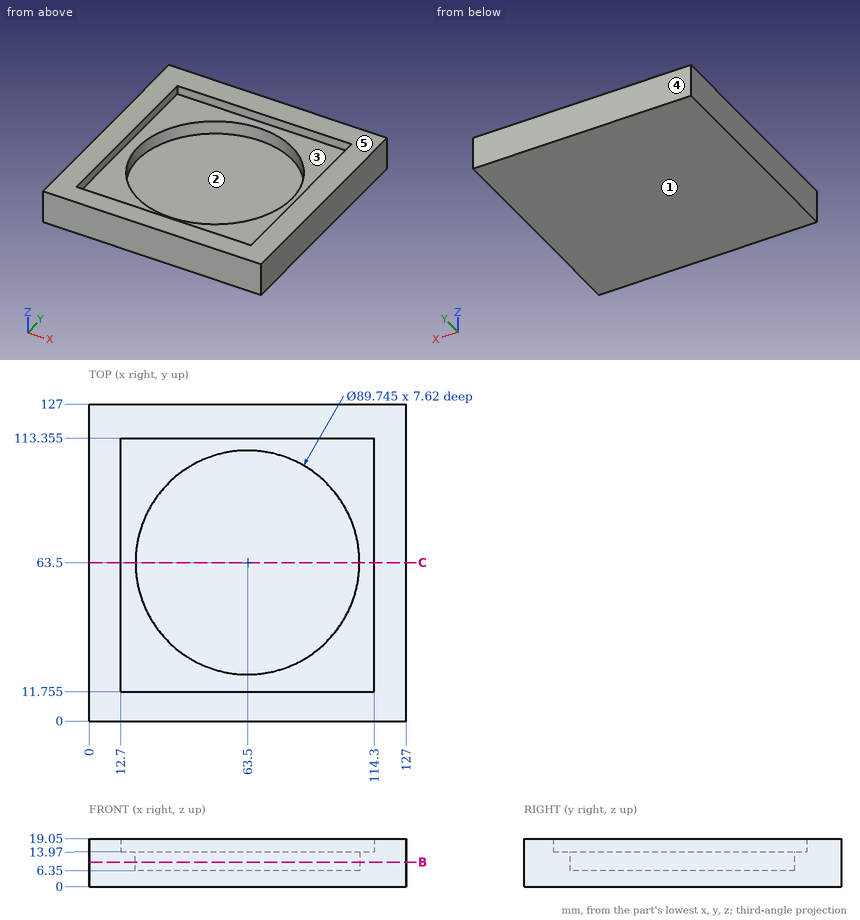
Answer from the drawing. Dimensions are ordinates in mm from the lowest x, y and z of the part. A direction names the side the tool comes from. Coordinates: 2 decimals unless noted, no trailing zeros. Write each loop counter-clockwise with the first axis right and the second up, starting at its lowest first coordinate (ties: lowest second). Pieces come first, ordered by that corner, then holes. Notation, with made-up numbers: (18.25, 33.25) - (27.25, 33.25) arc R32 ccw to (27.25, 60.25) - close; hole circle Ø8 at (41, -38.5). An arc over 180 degrees is marked (long way). Answer as CSV lines item,"result".
1. Find section B-B (z = 9.75). Give the vertices of the cut face in (x, y) (1 decimal).
Computed values:
outline,"(0, 0) - (127, 0) - (127, 127) - (0, 127) - close; hole circle Ø89.7 at (63.5, 63.5)"
2. Find section C-C (y = 63.5). Give the vertices of the cut face in (x, z), plus the area to 3 significant figures.
Computed values:
outline,"(0, 0) - (127, 0) - (127, 19.05) - (114.3, 19.05) - (114.3, 13.97) - (108.37, 13.97) - (108.37, 6.35) - (18.63, 6.35) - (18.63, 13.97) - (12.7, 13.97) - (12.7, 19.05) - (0, 19.05) - close"
area,"1,220 mm²"
3. A tool of negligible diameter and unlimited length cuts with its end or side. For the marked faces 1 and 2, from which of +Z, -Z, +X, -X, +Y, -Y can it reach the whole face along a straight path? Write none if from no direction.
Computed values:
face 1,"-Z, +X, -X, +Y, -Y"
face 2,"+Z"
4. Given P1, Ø2, axis at x = 41, y = 66.5, coming from the -Z side, flat-ended and moving along its own axis, determine where the tip first touches the part or whether it passes through.
Computed values:
P1,"stops at z = 0"
5. Determine the mould class of the marked faces 3, 4 and 5 for opening direction Y: +Y half, -Y half, draft (parallel to the pull), parting line (faces both ways), or undercut.
Computed values:
face 3,"undercut"
face 4,"+Y half"
face 5,"draft"
6. Straight lines are drawn through the part: line 1 (Y direction, x = 79.5, z = 17.75) (1 decimal); line 2 (X direction, y = 92, z = 15.5); line 3 (Z direction, x = 61, y = 24). For each, find the intervals that lie inside material, in ascending order. Write a range as [from, to].
Computed values:
line 1,"y = [0, 11.8], [113.4, 127]"
line 2,"x = [0, 12.7], [114.3, 127]"
line 3,"z = [0, 6.35]"
